Geometry: final body of the model. Coordinates: model frame, mm. Give positions to 0.01 mm unless a question says otherwise; leave off trailing zeros. Write each loop counter-clockwise with the first axis right and the second up, starting at its lowest first coordinate (ties: lowest second). Pieces come first, ordered by that corner, then holes. Notation, with made-up numbers: (53.5, 17) -> (71.5, 17) arc R21 ccw to (71.5, 27) -> close; hole circle Ø4 at (75, 16). An arc over 180 degrees is marked (long way). Answer in a Markdown table with one row per item. Add a question column.
Item 1: Section query B-B on x = -22.5. Output: boundary loops of the cut face in (y, z).
Item 2: Material intervals for probe 1 along X at (y, z) = (41.5, 25); probe 2 along X at (y, z) = (15, -34.5); probe 3 along Z at (x, y) = (19.5, 66.5), sorted ascending. Write a range as from..to.
Item 3: First-contact query: P1, Ø4, axis at x = -50, y = 23.5, coming from the -Z side; P2, Ø5, axis at x = -16.5, y = 31, coming from the +Z side; P3, Ø10, axis at y = 35.5, z = -1.5, coming from the +X side. Flat tips, straight axial feed; report the tip coordinate or a pass-through.
Item 4: Section query C-C on x = 0. Output: boundary loops of the cut face in (y, z).
Item 5: Section query D-D on y = 19. Output: boundary loops of the cut face in (x, z), plus the area to 3 significant figures.
Item 6: Section query A-A on z = 0. Output: boundary loops of the cut face in (x, y), plus the area to 3 significant figures.
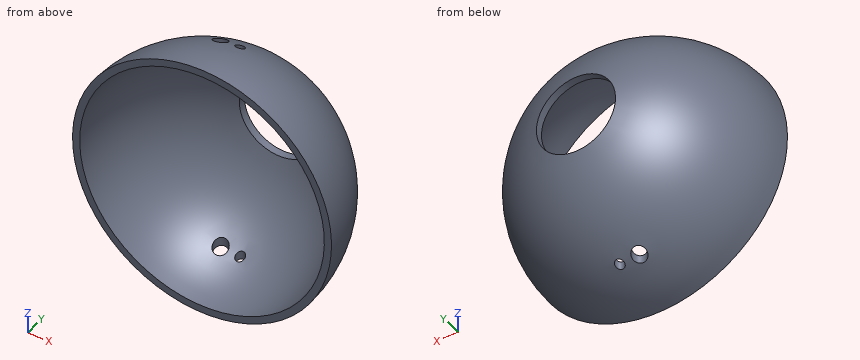
```python
from build123d import *

# Parameters (mm, degrees)
CUT_EXTRUDE5_DEPTH      = 154.439727581
CUT_EXTRUDE5_DEPTH_BACK = 154.439727581
SKETCH7_R               = 3.15
SKETCH7_R_2             = 5


with BuildPart() as part:
    # Sketch1 → Revolve1 (revolve)
    with BuildSketch(Plane.XY, mode=Mode.PRIVATE) as revolve1_sk:
        with BuildLine():
            Line((85, 0), (90, 0))
            ThreePointArc((90, 0), (72.715197861, 53.033008589), (27.5, 85.695682505))
            Line((27.5, 85.695682505), (27.5, 80.428539711))
            ThreePointArc((27.5, 80.428539711), (69.14658343, 49.434299833), (85, 0))
        make_face()
    revolve(revolve1_sk.sketch.rotate(Axis((0, 188.683155316, 0), (0, -1, 0)), 90), axis=Axis((0, 188.683155316, 0), (0, -1, 0)))

    # Sketch7 → Cut-Extrude5 (cut, two sides: drawn at the far end of the back side and taken through both)
    with BuildSketch(Plane.XY.offset(-CUT_EXTRUDE5_DEPTH_BACK)):
        with Locations(Location((0, 39.840172705, 0), (0, 0, 269.999999991))):
            Circle(SKETCH7_R)
        with Locations(Location((-13.579797877, 39.840172705, 0), (0, 0, 207.021474241))):
            Circle(SKETCH7_R_2)
    extrude(amount=CUT_EXTRUDE5_DEPTH + CUT_EXTRUDE5_DEPTH_BACK, mode=Mode.SUBTRACT)


solid = part.part
```
Findings below:
| question | item | result |
|---|---|---|
| 1 | outline | (0, -87.14) arc R87.14 ccw to (85.7, -15.81) -> (80.43, -15.81) arc R81.97 cw to (0, -81.97) -> close; (0, 81.97) arc R81.97 cw to (80.43, 15.81) -> (85.7, 15.81) arc R87.14 ccw to (0, 87.14) -> close |
| 2 | probe 1 | x = -75.85..-69.84, 69.84..75.85 |
| 2 | probe 2 | x = -81.76..-76.22, 76.22..81.76 |
| 2 | probe 3 | z = -57.42..-49.22, 49.22..57.42 |
| 3 | P1 | stops at z = -72.56 |
| 3 | P2 | stops at z = 83.88 |
| 3 | P3 | stops at x = 84.66 |
| 4 | outline | (0, -90) arc R90 ccw to (36.69, -82.18) -> (36.69, -76.67) arc R85 cw to (0, -85) -> close; (0, 85) arc R85 cw to (36.69, 76.67) -> (36.69, 82.18) arc R90 ccw to (0, 90) -> close; (42.99, -79.07) arc R90 ccw to (85.7, -27.5) -> (80.43, -27.5) arc R85 cw to (42.99, -73.33) -> close; (42.99, 73.33) arc R85 cw to (80.43, 27.5) -> (85.7, 27.5) arc R90 ccw to (42.99, 79.07) -> close |
| 5 | outline | circle Ø175.94 at (0, 0); hole circle Ø165.7 at (0, 0) |
| 5 | area | 2,750 mm^2 |
| 6 | outline | (-90, 0) -> (-85, 0) arc R85 cw to (-27.5, 80.43) -> (-27.5, 85.7) arc R90 ccw to start; (27.5, 80.43) arc R85 cw to (85, 0) -> (90, 0) arc R90 ccw to (27.5, 85.7) -> close |
| 6 | area | 1,090 mm^2 |
